Here's the drawing with two shaded views (mm, measured from the low corner). I have some questions. A direction names the side the tool comes from. Round coordinates to 2 decimals unless told otherwise and drop trailing zeros. Order: outer loops, then holes, each group sorted by start corner. A loop starts at its lowest first (then second) coordinate and runs counter-clockwise, first axis right, second up. Notation, with made-up numbers: (45.5, 49) -> (74.5, 49) arc R4 cw to (74.5, 53) -> close; hole circle Ø5 at (34, 17). An arc over 180 degrees is marked (long way). Answer in a Markdown table with one row per item.
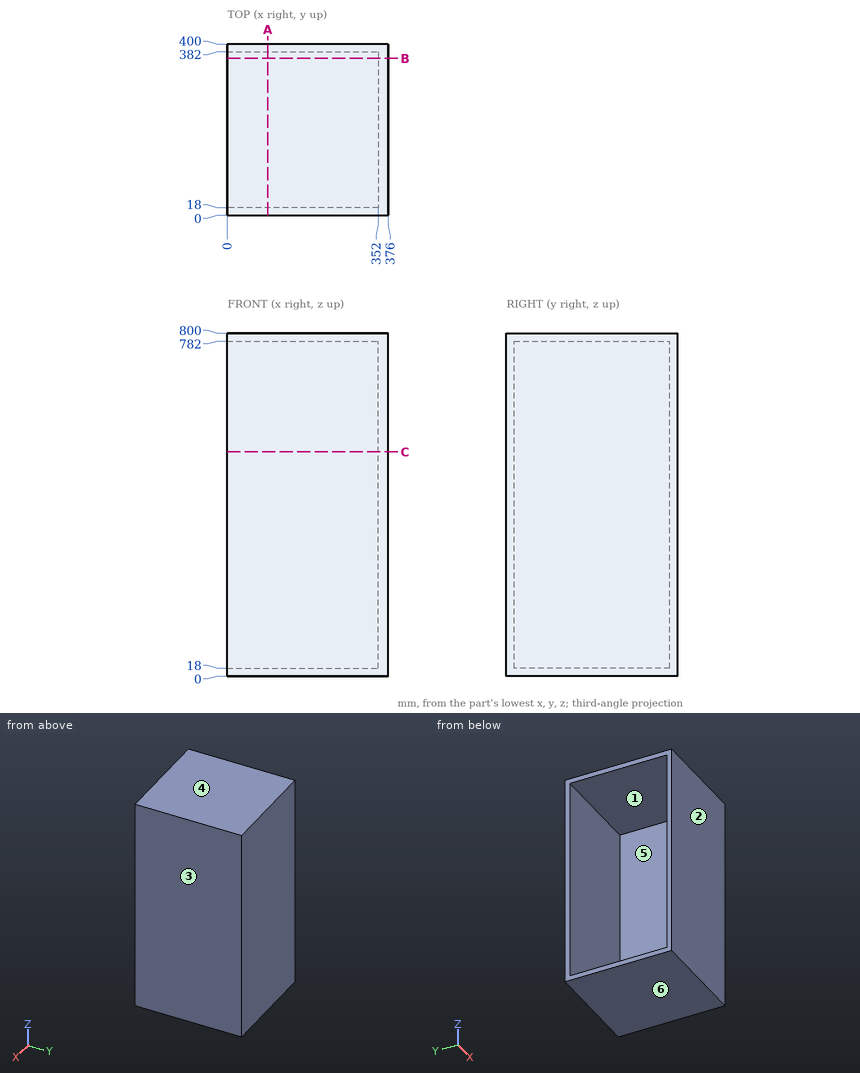
1. Suppose I cut it at B-B on y = 366.5. Write out the boundary of the cut face in (x, z), then the cut area to 3 significant figures.
Numbers:
| item | result |
|---|---|
| outline | (0, 0) -> (376, 0) -> (376, 800) -> (0, 800) -> (0, 782) -> (352, 782) -> (352, 18) -> (0, 18) -> close |
| area | 31,900 mm2 |
2. For pin 1 Ø4 at (y, z) = (127, 461) entering from -X; pin 2 Ø1 at (x, y) = (329.5, 183.5) entering from -Z, each with a flat end and sliding along its axis, tell me the tip position at first contact or that it passes through.
Numbers:
| item | result |
|---|---|
| pin 1 | stops at x = 352 |
| pin 2 | stops at z = 0 |
3. Suppose I cut it at A-A on x = 94.5. Write out the boundary of the cut face in (y, z).
Numbers:
| item | result |
|---|---|
| outline | (0, 0) -> (400, 0) -> (400, 800) -> (0, 800) -> close; hole (18, 18) -> (382, 18) -> (382, 782) -> (18, 782) -> close |
4. Please list where these lines run through material, in increasing order: line 1 along Z through (x, y) = (252.5, 177); line 2 along Y through (x, z) = (162, 309.5); line 3 along X through (y, z) = (90, 732.5).
Numbers:
| item | result |
|---|---|
| line 1 | z = 0 to 18, 782 to 800 |
| line 2 | y = 0 to 18, 382 to 400 |
| line 3 | x = 352 to 376 |
5. We'd pull the mould along Z, two halves only. Please class the marked faces 3, 4, 5 and 6: released by +Z, released by -Z, zero draft, split by the parting line, or undercut.
Numbers:
| item | result |
|---|---|
| face 3 | zero draft |
| face 4 | released by +Z |
| face 5 | undercut |
| face 6 | released by -Z |
6. Suppose I cut it at C-C on z = 523.5. Write out the boundary of the cut face in (x, y), then the cut area to 3 significant figures.
Numbers:
| item | result |
|---|---|
| outline | (0, 0) -> (376, 0) -> (376, 400) -> (0, 400) -> (0, 382) -> (352, 382) -> (352, 18) -> (0, 18) -> close |
| area | 22,300 mm2 |
7. For the marked faces 1 and 2, which set-ups out of +Z, -Z, +X, -X, +Y, -Y let a thin tool reach every point of the face, with its end or its side?
Numbers:
| item | result |
|---|---|
| face 1 | -X |
| face 2 | +Z, -Z, +X, -X, -Y |
